Geometry check sheet. Reference: the model listing, model coordinates, mm. Face numbers are marked on the shaded views. A direction names the side the tool comes from. Round coordinates to 2 decimals unless told otherwise and drop trailing zeros. Write each loop counter-clockwise with the first axis right and the second up, starting at its lowest first coordinate (ties: lowest second). Pieces come first, ordered by that corner, then holes. Notation, with made-up numbers: M 48,-20.75 L 91,-20.75 A20 cw 91,2.25 Z; hole C 63,1 d2. An arc over 180 degrees is marked long. One line per item, written item: value. Start each with the question number.
1. Access from +Z, -Z, +X, -X, +Y, -Y to the whole of each face (thin tool, end or side, straight path). Record for the marked faces 1, 2 and 3.
2. Section check A-A (x = -81). Record the boundary of the cut face in (y, z), and give its area (3 significant figures).
3. Scan lines: probe 1 along Y at (x, z) = (-73.5, 104.5); probe 2 along Z at (x, y) = (-14, 8). Record each from-to range of solid material in increasing order. Write a range as [from, to].
4. Section check C-C (z = 12.5). Record the boundary of the cut face in (x, y).
5. Section check B-B (y = 29.5). Record the boundary of the cut face in (x, z), and give its area (3 significant figures).
6. Depth check by flat-ended pin: P1, Ø12, axis at x = -34.5, z = 102, coming from the +Y side; P2, Ø2, axis at x = -9.5, z = 46.5, coming from the -Y side; P3, Ø0.6, axis at y = 4.5, z = 76.5, coming from the -X side. Enter the tip coordinate at first touch or a pass-through.
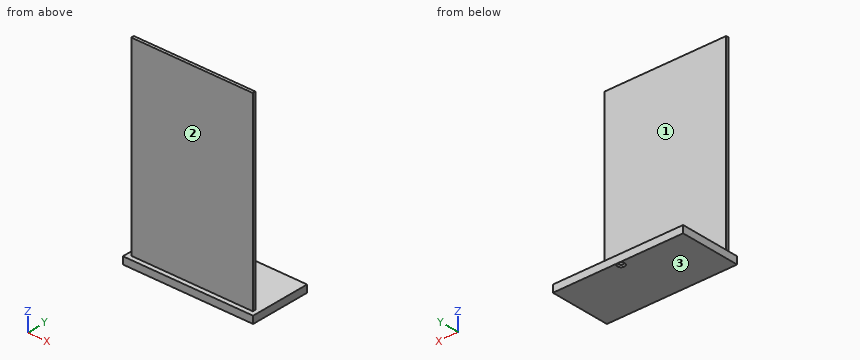
from build123d import *

# Parameters (mm, degrees)
SKETCH_W         = 90
SKETCH_H         = 42
PAD_DEPTH        = 5
SKETCH001_W      = 84
SKETCH001_H      = 2
PAD001_DEPTH     = 131.5
HOLE_D           = 3.2
HOLE_DEPTH       = 5
HOLE_CSINK_D     = 5
HOLE_CSINK_ANGLE = 90
HOLE_TIPS_R      = 1.6


with BuildPart() as part:
    # Sketch → Pad (new body)
    with BuildSketch(Plane.XY):
        with Locations((-45, 21)):
            Rectangle(SKETCH_W, SKETCH_H)
    extrude(amount=PAD_DEPTH)

    # Sketch001 (on Face6 of Pad) → Pad001 (join)
    with BuildSketch(Plane.XY.offset(5)):
        with Locations((-45.053107, 4.193032)):
            Rectangle(SKETCH001_W, SKETCH001_H)
    extrude(amount=PAD001_DEPTH)

    # Hole
    with Locations(Plane(origin=(0, 0, 0), x_dir=(1, 0, 0), z_dir=(0, 0, -1))):
        with Locations((-45.039894, -39.57151)):
            CounterSinkHole(HOLE_D / 2, HOLE_CSINK_D / 2, depth=HOLE_DEPTH, counter_sink_angle=HOLE_CSINK_ANGLE)

    # Hole tips → Hole tip 1 section 0
    with BuildSketch(Plane(origin=(0, 0, 5), x_dir=(1, 0, 0), z_dir=(0, 0, -1)), mode=Mode.PRIVATE) as hole_tip_1_s0:
        with Locations((-45.039894, -39.57151)):
            Circle(HOLE_TIPS_R)
    loft([hole_tip_1_s0.sketch, Vertex(-45.039894, 39.57151, 5.961377)], mode=Mode.SUBTRACT)


solid = part.part
Result sheet:
1. face 1: +Z, +X, -X, +Y
1. face 2: +Z, +X, -X, -Y
1. face 3: -Z, +X, -X, +Y, -Y
2. outline: M 0,0 L 42,0 L 42,5 L 5.19,5 L 5.19,136.5 L 3.19,136.5 L 3.19,5 L 0,5 Z
2. area: 473 mm2
3. probe 1: y = [3.19, 5.19]
3. probe 2: z = [0, 5]
4. outline: M -87.05,3.19 L -3.05,3.19 L -3.05,5.19 L -87.05,5.19 Z
5. outline: M -90,0 L 0,0 L 0,5 L -90,5 Z
5. area: 450 mm2
6. P1: stops at y = 5.19
6. P2: stops at y = 3.19
6. P3: stops at x = -87.05
